from build123d import *

# Parameters (mm, degrees)
SKETCH1_R               = 62
BOSS_EXTRUDE1_DEPTH     = 5
SKETCH2_R               = 2
CUT_EXTRUDE1_DEPTH      = 5
CIRPATTERN1_COUNT       = 2
CIRPATTERN1_ANGLE       = 120
MIRROR1_COPY_1_SKETCH_R = 2
MIRROR1_COPY_1_DEPTH    = 5
SKETCH5_R               = 32.5
CUT_EXTRUDE2_DEPTH      = 10


with BuildPart() as part:
    # Sketch1 → Boss-Extrude1 (new body)
    with BuildSketch(Plane(origin=(0, 0, 0), x_dir=(1, 0, 0), z_dir=(0, 1, 0))):
        with Locations(Location((0, 0, 0), (0, 0, 270))):
            Circle(SKETCH1_R)
    extrude(amount=BOSS_EXTRUDE1_DEPTH)

    # Sketch2 → Cut-Extrude1 (cut)
    with BuildSketch(Plane(origin=(0, 5, 0), x_dir=(1, 0, 0), z_dir=(0, 1, 0))):
        with Locations(Location((0, 49.5, 0), (0, 0, 270))):
            Circle(SKETCH2_R)
    cut_extrude1 = extrude(amount=-CUT_EXTRUDE1_DEPTH, mode=Mode.SUBTRACT)

    # CirPattern1: Cut-Extrude1 ×2 about axis
    cirpattern1_axis = Axis((0, 5, 0), (0, 1, 0))
    for i in range(1, CIRPATTERN1_COUNT):
        add(cut_extrude1.rotate(cirpattern1_axis, i * CIRPATTERN1_ANGLE / (CIRPATTERN1_COUNT - 1)), mode=Mode.SUBTRACT)

    # Mirror1: Cut-Extrude1 across plane
    add(cut_extrude1.mirror(Plane(origin=(0, 0, 0), x_dir=(-0.49999999999999806, 0, 0.8660254037844398), z_dir=(-0.8660254037844398, 0, -0.49999999999999806))), mode=Mode.SUBTRACT)

    # Mirror1 copy 1 sketch → Mirror1 copy 1 (cut)
    with BuildSketch(Plane(origin=(0, 5, 0), x_dir=(1, 0, 0), z_dir=(0, 1, 0))):
        with Locations((0, -49.5)):
            Circle(MIRROR1_COPY_1_SKETCH_R)
    extrude(amount=-MIRROR1_COPY_1_DEPTH, mode=Mode.SUBTRACT)

    # Sketch5 → Cut-Extrude2 (cut)
    with BuildSketch(Plane.XZ):
        with Locations(Location((0, 0, 0), (0, 0, 270))):
            Circle(SKETCH5_R)
    extrude(amount=-CUT_EXTRUDE2_DEPTH, mode=Mode.SUBTRACT)


solid = part.part
The model under review builds one solid part; all positions refer to its coordinate system, in mm. Give positions to 0.01 mm unless a question says otherwise; leave off trailing zeros. Write each loop counter-clockwise with the first axis right and the second up, starting at its lowest first coordinate (ties: lowest second). Pieces come first, ordered by that corner, then holes.
1. Add section B-B, the plane x = -3.5. Write out the cut boundary in (y, z).
2. Add section C-C, the plane y = 2. Write out the cut boundary in (x, z).
3. Wall thickness on L1, parallel to X at y = 2.65, z = -24.75; L2, parallel to X at y = 3.15, z = 49.5; L3, parallel to Z at x = 17.5, y = 3.1: over which ranges is each line inside the solid? List them lowest first.
4. Add section A-A, the plane z = 0. Write out the cut boundary in (x, y), plus the area to 3 significant figures.
5. Draft analysis for pull direction X (two halves, no side actions). For faces 1 (the cylindrical face through (-44.82, 2.54, 24.32)), 2 (the flat face through (-27, 5, 27)), 3 (the cylindrical face through (61.472, 2.465, -8.071)), state which applies: +X half, -X half, draft (parallel to the pull), parting line (faces both ways), or undercut.
6. For P1, Ø1.5, axis at y = 1, z = -41.5, coming from the -X side; P2, Ø1.5, axis at x = -5, y = 3.5, coming from the +Z side; P3, Ø1.5, axis at x = -39, y = 2, coming from the -Z side, all flat-tipped, find the tip position at first contact; note any pin that passes through.
7. Add section D-D, the plane z = -41. Write out the cut boundary in (x, y).
Worked answers:
1. outline: (0, -61.9) - (5, -61.9) - (5, -32.31) - (0, -32.31) - close; (0, 32.31) - (5, 32.31) - (5, 61.9) - (0, 61.9) - close
2. outline: circle Ø124 at (0, 0); hole circle Ø4 at (-42.87, 24.75); hole circle Ø65 at (0, 0); hole circle Ø4 at (0, -49.5); hole circle Ø4 at (0, 49.5); hole circle Ø4 at (42.87, -24.75)
3. L1: x = -56.85 to -21.06, 21.06 to 40.87, 44.87 to 56.85
3. L2: x = -37.33 to -2, 2 to 37.33
3. L3: z = -59.48 to -27.39, 27.39 to 59.48
4. outline: (-62, 0) - (-32.5, 0) - (-32.5, 5) - (-62, 5) - close; (32.5, 0) - (62, 0) - (62, 5) - (32.5, 5) - close
4. area: 295 mm2
5. face 1: undercut
5. face 2: draft
5. face 3: parting line
6. P1: stops at x = -46.73
6. P2: stops at z = 61.85
6. P3: stops at z = -48.79
7. outline: (-46.51, 0) - (46.51, 0) - (46.51, 5) - (-46.51, 5) - close
